Drawing for the job (mm, zero at the part's lowest x, y, z). Round coordinates to 2 decimals unless told otherwise and drop trailing zeros. Loops run counter-clockwise (first coordinate to the right, second up) from the corner with the lowest first, then second, coordinate; pieces in that order, holes last. Notation, with made-up numbers: M 13,72.5 L 25,72.5 A26 ccw 25,89.5 Z; hole C -35.75,62 d3. An arc over 180 degrees is marked long. Answer in a Markdown table with one row per item.
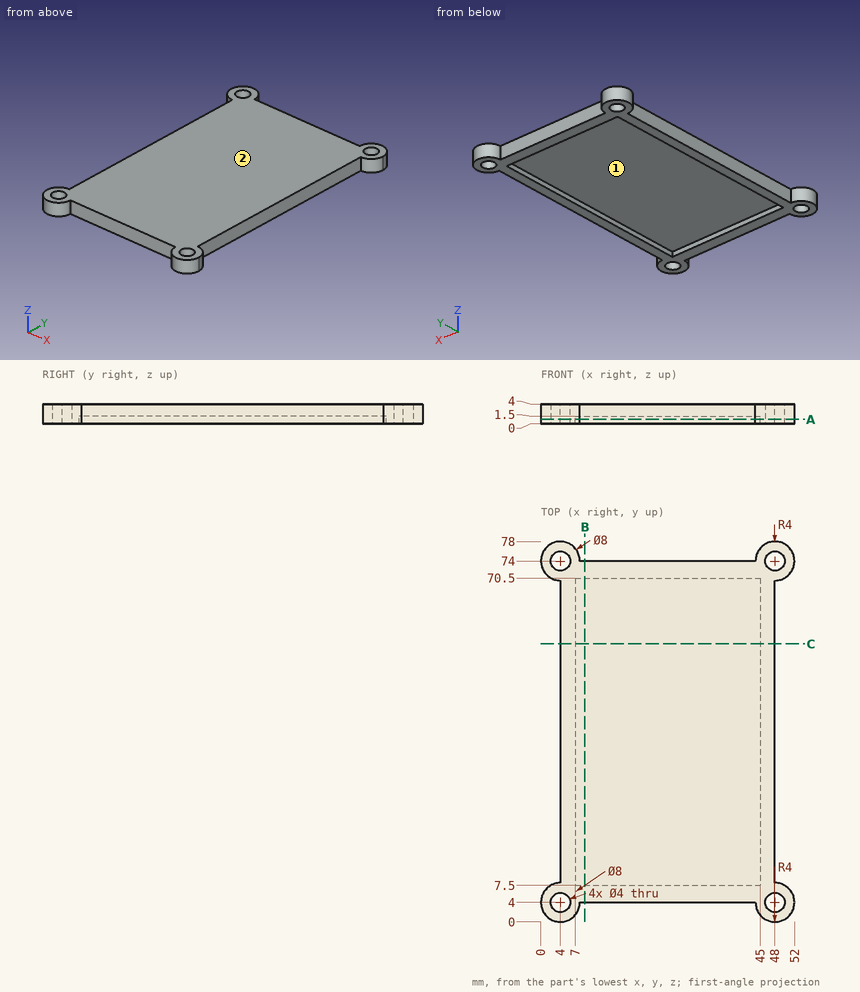
1. Saw through at C-C (y = 57). Write the cut outline in (x, z), and give its area (3 significant figures).
Verdict:
| item | result |
|---|---|
| outline | M 4,0 L 7,0 L 7,1.5 L 45,1.5 L 45,0 L 48,0 L 48,4 L 4,4 Z |
| area | 119 mm² |
2. Mould opens along Y. For the marked faces 1 and 2 say: +Y half, -Y half, draft (parallel to the pull), parting line (faces both ways), or undercut.
Verdict:
| item | result |
|---|---|
| face 1 | undercut |
| face 2 | draft |
3. Pin check, flat tips, straight feed: pin 1 (3.5 mm diameter, centred on x = 48, y = 74, fed in from -Z); pin 2 (2 mm diameter, centred on y = 27.5, z = 2.5, fed in from +X); pin 3 (1 mm diameter, centred on x = 31.5, z = 1.5, fed in from +Y); pin 4 (0.8 mm diameter, centred on x = 34.5, z = 1, fed in from -Y). Stop position of each tip, or through.
Verdict:
| item | result |
|---|---|
| pin 1 | passes through |
| pin 2 | stops at x = 48 |
| pin 3 | stops at y = 74 |
| pin 4 | stops at y = 4 |
4. Saw through at B-B (x = 9). Write the cut outline in (y, z), and give its area (4 significant figures).
Verdict:
| item | result |
|---|---|
| outline | M 4,0 L 7.5,0 L 7.5,1.5 L 70.5,1.5 L 70.5,0 L 74,0 L 74,4 L 4,4 Z |
| area | 185.5 mm² |
5. Wall check: probe 1 along X at (y, z) = (16, 1); probe 2 along Y at (x, z) = (30, 0.3); probe 3 along Z at (x, y) = (25.5, 23.5). Give the ranges that are in metal, low to high.
Verdict:
| item | result |
|---|---|
| probe 1 | x = 4 to 7, 45 to 48 |
| probe 2 | y = 4 to 7.5, 70.5 to 74 |
| probe 3 | z = 1.5 to 4 |
6. Saw through at A-A (z = 0.85). Write the cut outline in (x, y), and give its area (3 significant figures).
Verdict:
| item | result |
|---|---|
| outline | M 4,8 A4 ccw long 8,4 L 44,4 A4 ccw long 48,8 L 48,70 A4 ccw long 44,74 L 8,74 A4 ccw long 4,70 Z; hole C 4,4 d4; hole C 4,74 d4; hole M 7,7.5 L 45,7.5 L 45,70.5 L 7,70.5 Z; hole C 48,4 d4; hole C 48,74 d4 |
| area | 787 mm² |
